```python
from build123d import *

# Parameters (mm, degrees)
F0_R      = 72.5
F0_R_2    = 58.5
F1_DEPTH  = 10
F3_DEPTH  = 10.001
F5_DEPTH  = 5
F7_DEPTH  = 2
F8_SIZE   = 3
F9_R      = 5
F10_R     = 2
F11_W     = 21.5406592285
F11_H     = 1
F11_W_2   = 1
F11_H_2   = 21.5406592285
F12_DEPTH = 10


with BuildPart() as f1:
    # F0 (on Top) → F1 (new body)
    with BuildSketch(Plane.XY):
        Circle(F0_R)
        with BuildLine():
            ThreePointArc((2, -66.5), (0, -68.5), (-2, -66.5))
            Line((-2, -66.5), (-2, -64.5))
            ThreePointArc((-2, -64.5), (0, -62.5), (2, -64.5))
            Line((2, -64.5), (2, -66.5))
        make_face(mode=Mode.SUBTRACT)
        with BuildLine():
            Line((-65.5, 2), (-64.5, 2))
            ThreePointArc((-64.5, 2), (-63.0857864376, 1.4142135624), (-62.5, 0))
            ThreePointArc((-62.5, 0), (-63.0857864376, -1.4142135624), (-64.5, -2))
            Line((-64.5, -2), (-65.5, -2))
            Line((-65.5, -2), (-66.5, -2))
            ThreePointArc((-66.5, -2), (-68.5, 0), (-66.5, 2))
            Line((-66.5, 2), (-65.5, 2))
        make_face(mode=Mode.SUBTRACT)
        Circle(F0_R_2, mode=Mode.SUBTRACT)
        with BuildLine():
            ThreePointArc((66.5, 2), (67.9142135624, 1.4142135624), (68.5, 0))
            ThreePointArc((68.5, 0), (67.9142135624, -1.4142135624), (66.5, -2))
            Line((66.5, -2), (64.5, -2))
            ThreePointArc((64.5, -2), (62.5, 0), (64.5, 2))
            Line((64.5, 2), (66.5, 2))
        make_face(mode=Mode.SUBTRACT)
        with BuildLine():
            ThreePointArc((-2, 66.5), (0, 68.5), (2, 66.5))
            Line((2, 66.5), (2, 64.5))
            ThreePointArc((2, 64.5), (0, 62.5), (-2, 64.5))
            Line((-2, 64.5), (-2, 66.5))
        make_face(mode=Mode.SUBTRACT)
    extrude(amount=F1_DEPTH)

    # F2 (on face) → F3 (cut, through all)
    with BuildSketch(Plane.XY.offset(10)):
        Polygon((39.5494049015, -60.7626083371), (40.6586399182, -61.8718433538), (61.8718433538, -40.6586399182), (60.7626083371, -39.5494049015), align=None)
        with BuildLine():
            ThreePointArc((39.5494049015, -60.7626083371), (45.6549558742, -56.319401667), (51.2652415538, -51.2652417182))
            ThreePointArc((51.2652415538, -51.2652417182), (56.3194015937, -45.6549559645), (60.7626083371, -39.5494049015))
            Line((60.7626083371, -39.5494049015), (39.5494049015, -60.7626083371))
        make_face()
    extrude(amount=-F3_DEPTH, mode=Mode.SUBTRACT)

    # F4 (on face) → F5 (cut)
    with BuildSketch(Plane.XY.offset(10)):
        Polygon((55.6760094304, -34.4628059948), (50.5894105236, -29.376207088), (29.376207088, -50.5894105236), (34.4628059948, -55.6760094304), align=None)
    extrude(amount=-F5_DEPTH, mode=Mode.SUBTRACT)

    # F6 (on face) → F7 (cut)
    with BuildSketch(Plane.XY.offset(10)):
        with BuildLine():
            ThreePointArc((-65, -5.0251865637), (-61.7565056431, -3.3895058637), (-60.45, 0))
            ThreePointArc((-60.45, 0), (-61.7565056431, 3.3895058637), (-65, 5.0251865637))
            ThreePointArc((-65, 5.0251865637), (-69.55, 0), (-65, -5.0251865637))
        make_face()
        with BuildLine():
            ThreePointArc((-65, 5.0251865637), (-61.7565056431, 3.3895058637), (-60.45, 0))
            ThreePointArc((-60.45, 0), (-61.7565056431, -3.3895058637), (-65, -5.0251865637))
            ThreePointArc((-65, -5.0251865637), (-61.1104941363, -3.7434943569), (-59.45, 0))
            ThreePointArc((-59.45, 0), (-61.1104941363, 3.7434943569), (-65, 5.0251865637))
        make_face()
        with BuildLine():
            ThreePointArc((-65, -5.0251865637), (-69.55, 0), (-65, 5.0251865637))
            ThreePointArc((-65, 5.0251865637), (-70.55, 0), (-65, -5.0251865637))
        make_face()
        with BuildLine():
            ThreePointArc((5.0251865637, 65), (5.0437928262, 65.249692336), (5.05, 65.5))
            ThreePointArc((5.05, 65.5), (-0.250307664, 70.5437928262), (-5.0251865637, 65))
            ThreePointArc((-5.0251865637, 65), (0, 69.55), (5.0251865637, 65))
        make_face()
        with BuildLine():
            ThreePointArc((5.0251865637, 65), (0, 69.55), (-5.0251865637, 65))
            ThreePointArc((-5.0251865637, 65), (0, 60.45), (5.0251865637, 65))
        make_face()
        with BuildLine():
            ThreePointArc((5.0251865637, 65), (0, 60.45), (-5.0251865637, 65))
            ThreePointArc((-5.0251865637, 65), (-0.250307664, 59.4562071738), (5.05, 64.5))
            ThreePointArc((5.05, 64.5), (5.0437928262, 64.750307664), (5.0251865637, 65))
        make_face()
        with BuildLine():
            ThreePointArc((65, -5.0251865637), (68.8895058637, -3.7434943569), (70.55, 0))
            ThreePointArc((70.55, 0), (68.8895058637, 3.7434943569), (65, 5.0251865637))
            ThreePointArc((65, 5.0251865637), (68.2434943569, 3.3895058637), (69.55, 0))
            ThreePointArc((69.55, 0), (68.2434943569, -3.3895058637), (65, -5.0251865637))
        make_face()
        with BuildLine():
            ThreePointArc((69.55, 0), (68.2434943569, 3.3895058637), (65, 5.0251865637))
            ThreePointArc((65, 5.0251865637), (60.45, 0), (65, -5.0251865637))
            ThreePointArc((65, -5.0251865637), (68.2434943569, -3.3895058637), (69.55, 0))
        make_face()
        with BuildLine():
            ThreePointArc((65, -5.0251865637), (60.45, 0), (65, 5.0251865637))
            ThreePointArc((65, 5.0251865637), (59.45, 0), (65, -5.0251865637))
        make_face()
        with BuildLine():
            ThreePointArc((-5.0251865637, -65), (-0.250307664, -70.5437928262), (5.05, -65.5))
            ThreePointArc((5.05, -65.5), (5.0437928262, -65.249692336), (5.0251865637, -65))
            ThreePointArc((5.0251865637, -65), (0, -69.55), (-5.0251865637, -65))
        make_face()
        with BuildLine():
            ThreePointArc((-5.0251865637, -65), (0, -69.55), (5.0251865637, -65))
            ThreePointArc((5.0251865637, -65), (0, -60.45), (-5.0251865637, -65))
        make_face()
        with BuildLine():
            ThreePointArc((-5.0251865637, -65), (0, -60.45), (5.0251865637, -65))
            ThreePointArc((5.0251865637, -65), (5.0437928262, -64.750307664), (5.05, -64.5))
            ThreePointArc((5.05, -64.5), (-0.250307664, -59.4562071738), (-5.0251865637, -65))
        make_face()
    extrude(amount=-F7_DEPTH, mode=Mode.SUBTRACT)

    # F8
    f8_edges = [f1.edges().sort_by_distance(p)[0] for p in [
        (41.365747, -41.365747, 5),
    ]]
    chamfer(f8_edges, length=F8_SIZE)

    # F9
    f9_edges = [f1.edges().sort_by_distance(p)[0] for p in [
        (43.487067, -43.487067, 5),
    ]]
    fillet(f9_edges, radius=F9_R)

    # F10
    f10_edges = [f1.edges().sort_by_distance(p)[0] for p in [
        (55.676009, -34.462806, 7.5),
        (34.462806, -55.676009, 7.5),
    ]]
    fillet(f10_edges, radius=F10_R)

    # F11 (on face) → F12 (join)
    with BuildSketch(Plane.XY.offset(10)):
        with Locations((0, -58)):
            Rectangle(F11_W, F11_H)
        with Locations((58, 0)):
            Rectangle(F11_W_2, F11_H_2)
        with Locations((0, 58)):
            Rectangle(F11_W, F11_H)
        with Locations((-58, 0)):
            Rectangle(F11_W_2, F11_H_2)
    extrude(amount=-F12_DEPTH)


solid = f1.part
```
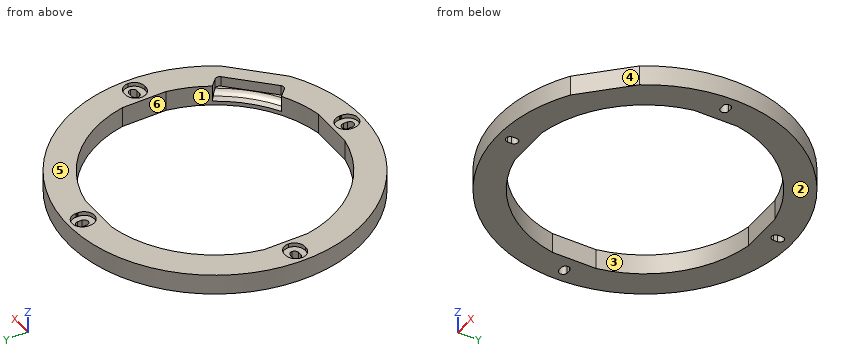
Here's how the part is built. I have some questions about the finished solid (model axes, mm). Face numbers are marked on the shaded views. A direction names the side the tool comes from. Coordinates: 2 decimals unless noted, no trailing zeros. Loops run counter-clockwise (first coordinate to the right, second up) from the corner with the lowest first, then second, coordinate; pieces in that order, holes last. Notation, with made-up numbers: (30, -7.75) - (79, -7.75) arc R21 ccw to (79, 19.25) - close; hole circle Ø9 at (-29, -32). An arc over 180 degrees is marked (long way). Return JSON: item names as keys, results as strings. Group by question number.
Item 1: We'd pull the mould along X, two halves only. Please class the marked faces 1, 2, 3 and 4: +X half, -X half, draft (parallel to the pull), parting line (faces both ways), or undercut.
Item 2: On a 3-axis mill with a long thin cutter (end or side, diameter ignored), from which of +Z, -Z, +X, -X, +Y, -Y can I reach the whole of each face in a straight line? I mean the marked faces 5 and 6. Say none if no direction works.
Item 3: If we section it at B-B on x = -27: Write out the boundary of the cut face in (y, z), and give its area (3 significant figures).
Item 4: If we section it at A-A on y = -7.5: Write out the boundary of the cut face in (x, z), and give its area (3 significant figures).
Item 5: I need wall thicknesses on line 1 (Y direction, x = 64.5, z = 9.45); line 2 (Y direction, x = -65.5, z = 8.5); line 3 (X direction, y = -6, z = 5). Which ranges of each line are inside material? Lowest first, please. Write a range as from..to.
Item 6: Will these pins go through, and if not, where does the flat tip stop? P1, Ø0.6, axis at y = 65, z = 2, coming from the -X side; P2, Ø5, axis at x = 0.5, y = 66, coming from the +Z side; P3, Ø0.6, axis at x = -66, z = 3, coming from the -Y side.
Calculated:
{
 "1": {"face 1": "undercut", "face 2": "draft", "face 3": "undercut", "face 4": "+X half"},
 "2": {"face 5": "+Z, +X, -X, +Y, -Y", "face 6": "+Z, -Z"},
 "3": {"outline": "(-67.28, 0) - (-51.9, 0) - (-51.9, 10) - (-67.28, 10) - close; (51.9, 0) - (67.28, 0) - (67.28, 10) - (51.9, 10) - close", "area": "308 mm^2"},
 "4": {"outline": "(-72.11, 0) - (-57.5, 0) - (-57.5, 10) - (-72.11, 10) - close; (57.5, 0) - (72.11, 0) - (72.11, 10) - (57.5, 10) - close", "area": "292 mm^2"},
 "5": {"line 1": "y = -33.11..-5.05, 5.05..33.11", "line 2": "y = -31.08..-5.05, 5.05..31.08", "line 3": "x = -72.25..-57.5, 57.5..72.25"},
 "6": {"P1": "stops at x = -32.71", "P2": "stops at z = 8", "P3": "stops at y = -30.66"}
}
